```python
from build123d import *

# Parameters (mm, degrees)
F0_R     = 140
F1_DEPTH = 15
F3_DEPTH = 15.001
F5_DEPTH = 15.001


with BuildPart() as f1:
    # F0 (on Top) → F1 (new body)
    with BuildSketch(Plane.XY):
        Circle(F0_R)
    extrude(amount=F1_DEPTH)

    # F2 (on face) → F3 (cut, through all)
    with BuildSketch(Plane.XY.offset(15)):
        with BuildLine():
            ThreePointArc((-107, 0), (-107.8642650828, 2.1068071491), (-109.9590909091, 2.9997210614))
            ThreePointArc((-109.9590909091, 2.9997210614), (-110, 0), (-109.9590909091, -2.9997210614))
            ThreePointArc((-109.9590909091, -2.9997210614), (-107.8642650828, -2.1068071491), (-107, 0))
        make_face()
        with BuildLine():
            ThreePointArc((-109.9590909091, -2.9997210614), (-110, 0), (-109.9590909091, 2.9997210614))
            ThreePointArc((-109.9590909091, 2.9997210614), (-113, 0), (-109.9590909091, -2.9997210614))
        make_face()
        with BuildLine():
            ThreePointArc((-2.9997210614, 109.9590909091), (0, 110), (2.9997210614, 109.9590909091))
            ThreePointArc((2.9997210614, 109.9590909091), (2.9999302645, 109.9795449791), (3, 110))
            ThreePointArc((3, 110), (-0.0204550209, 112.9999302645), (-2.9997210614, 109.9590909091))
        make_face()
        with BuildLine():
            ThreePointArc((-2.9997210614, 109.9590909091), (0, 107), (2.9997210614, 109.9590909091))
            ThreePointArc((2.9997210614, 109.9590909091), (0, 110), (-2.9997210614, 109.9590909091))
        make_face()
        with BuildLine():
            ThreePointArc((-2.9997210614, -109.9590909091), (0, -110), (2.9997210614, -109.9590909091))
            ThreePointArc((2.9997210614, -109.9590909091), (0, -107), (-2.9997210614, -109.9590909091))
        make_face()
        with BuildLine():
            ThreePointArc((3, -110), (2.9999302645, -109.9795449791), (2.9997210614, -109.9590909091))
            ThreePointArc((2.9997210614, -109.9590909091), (0, -110), (-2.9997210614, -109.9590909091))
            ThreePointArc((-2.9997210614, -109.9590909091), (-0.0204550209, -112.9999302645), (3, -110))
        make_face()
        with BuildLine():
            ThreePointArc((109.9590909091, -2.9997210614), (109.9897722518, -1.5), (110, 0))
            ThreePointArc((110, 0), (109.9897722518, 1.5), (109.9590909091, 2.9997210614))
            ThreePointArc((109.9590909091, 2.9997210614), (107, 0), (109.9590909091, -2.9997210614))
        make_face()
        with BuildLine():
            ThreePointArc((109.9590909091, 2.9997210614), (109.9897722518, 1.5), (110, 0))
            ThreePointArc((110, 0), (109.9897722518, -1.5), (109.9590909091, -2.9997210614))
            ThreePointArc((109.9590909091, -2.9997210614), (112.1068071491, -2.1357349172), (113, 0))
            ThreePointArc((113, 0), (112.1068071491, 2.1357349172), (109.9590909091, 2.9997210614))
        make_face()
    extrude(amount=-F3_DEPTH, mode=Mode.SUBTRACT)

    # F4 (on face) → F5 (cut, through all)
    with BuildSketch(Plane.XY.offset(15)):
        with BuildLine():
            Line((3.5355339059, -3.5355339059), (0, 0))
            Line((0, 0), (-3.5355339059, 3.5355339059))
            ThreePointArc((-3.5355339059, 3.5355339059), (-3.5355339059, -3.5355339059), (3.5355339059, -3.5355339059))
        make_face()
        with BuildLine():
            Line((-3.5355339059, 3.5355339059), (0, 0))
            Line((0, 0), (3.5355339059, -3.5355339059))
            ThreePointArc((3.5355339059, -3.5355339059), (4.6193976626, -1.9134171618), (5, 0))
            ThreePointArc((5, 0), (1.9134171618, 4.6193976626), (-3.5355339059, 3.5355339059))
        make_face()
        with BuildLine():
            ThreePointArc((-43.5355339059, 43.5355339059), (-43.5355339059, 36.4644660941), (-36.4644660941, 36.4644660941))
            Line((-36.4644660941, 36.4644660941), (-43.5355339059, 43.5355339059))
        make_face()
        with BuildLine():
            Line((-43.5355339059, 43.5355339059), (-36.4644660941, 36.4644660941))
            ThreePointArc((-36.4644660941, 36.4644660941), (-35.3806023374, 38.0865828382), (-35, 40))
            ThreePointArc((-35, 40), (-38.0865828382, 44.6193976626), (-43.5355339059, 43.5355339059))
        make_face()
        with BuildLine():
            ThreePointArc((-23.5355339059, 23.5355339059), (-23.5355339059, 16.4644660941), (-16.4644660941, 16.4644660941))
            Line((-16.4644660941, 16.4644660941), (-23.5355339059, 23.5355339059))
        make_face()
        with BuildLine():
            Line((-23.5355339059, 23.5355339059), (-16.4644660941, 16.4644660941))
            ThreePointArc((-16.4644660941, 16.4644660941), (-15.3806023374, 18.0865828382), (-15, 20))
            ThreePointArc((-15, 20), (-18.0865828382, 24.6193976626), (-23.5355339059, 23.5355339059))
        make_face()
        with BuildLine():
            ThreePointArc((45, -40), (41.9134171618, -35.3806023374), (36.4644660941, -36.4644660941))
            Line((36.4644660941, -36.4644660941), (43.5355339059, -43.5355339059))
            ThreePointArc((43.5355339059, -43.5355339059), (44.6193976626, -41.9134171618), (45, -40))
        make_face()
        with BuildLine():
            Line((43.5355339059, -43.5355339059), (36.4644660941, -36.4644660941))
            ThreePointArc((36.4644660941, -36.4644660941), (36.4644660941, -43.5355339059), (43.5355339059, -43.5355339059))
        make_face()
        with BuildLine():
            ThreePointArc((25, -20), (21.9134171618, -15.3806023374), (16.4644660941, -16.4644660941))
            Line((16.4644660941, -16.4644660941), (23.5355339059, -23.5355339059))
            ThreePointArc((23.5355339059, -23.5355339059), (24.6193976626, -21.9134171618), (25, -20))
        make_face()
        with BuildLine():
            Line((23.5355339059, -23.5355339059), (16.4644660941, -16.4644660941))
            ThreePointArc((16.4644660941, -16.4644660941), (16.4644660941, -23.5355339059), (23.5355339059, -23.5355339059))
        make_face()
    extrude(amount=-F5_DEPTH, mode=Mode.SUBTRACT)


solid = f1.part
```
Design review of the part built by this model. Coordinates are the model's own, in mm. Coordinates: 2 decimals unless noted, no trailing zeros. Order: outer loops, then holes, each group sorted by start corner. A loop starts at its lowest first (then second) coordinate and runs counter-clockwise, first axis right, second up.
1) Take a section at D-D, the plane x = -85.5. Give the boundary of the cut face in (y, z).
2) Take a section at A-A, the plane z = 12.75. State how many separate pieces and enclosed holes the cut face has, and give its area (3 significant figures).
3) Wall thickness on line 1 along X through (y, z) = (-40.5, 5.25); line 2 along X through (y, z) = (37.5, 11.75); line 3 along Y through (x, z) = (-44, 7.25): over which ranges is each line inside the solid? List them lowest first.
4) Take a section at C-C, the plane y = 49. Give the boundary of the cut face in (x, z).
5) Take a section at B-B, the plane x = 40. Give the boundary of the cut face in (y, z), and give its area (3 significant figures).
6) Clearance check with flat-ended pins moving along their axes: pin 1 (6 mm diameter, centred on x = 61, z = 6, fed in from -Y); pin 2 (3 mm diameter, centred on x = -11, z = 10, fed in from -Y); pin 3 (2 mm diameter, centred on x = -66.5, z = 3, fed in from +Y). State where each tip first meets the part, or that it passes through.
7) Mouldability with a two-part tool opening along Y and no side actions: class faces 1 (the cylindrical face through (-111.1, -85.19, 7.4)), 2 (the flat face through (-2, -29, 15)) as +Y half, -Y half, draft (parallel to the pull), parting line (faces both ways), or undercut.
Returned:
1. outline: (-110.86, 0) - (110.86, 0) - (110.86, 15) - (-110.86, 15) - close
2. separate pieces: 1
2. enclosed holes: 9
2. area: 61,100 mm2
3. line 1: x = -134.01 to 35.03, 44.97 to 134.01
3. line 2: x = -134.88 to -44.33, -35.67 to 134.88
3. line 3: y = -132.91 to 37, 43 to 132.91
4. outline: (-131.14, 0) - (131.14, 0) - (131.14, 15) - (-131.14, 15) - close
5. outline: (-134.16, 0) - (-45, 0) - (-45, 15) - (-134.16, 15) - close; (-35, 0) - (134.16, 0) - (134.16, 15) - (-35, 15) - close
5. area: 3,870 mm2
6. pin 1: stops at y = -127.42
6. pin 2: stops at y = -139.68
6. pin 3: stops at y = 123.73
7. face 1: parting line
7. face 2: draft
